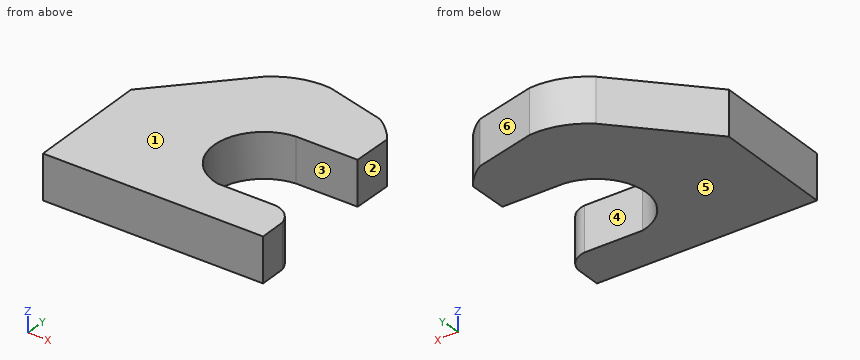
```python
from build123d import *

# Parameters (mm, degrees)
TABAN_FLAN_1_DEPTH         = 50
KES_EKSTR_ZYON1_DEPTH      = 585.997809561
KES_EKSTR_ZYON1_DEPTH_BACK = 585.997809561


# Sheet-metal steps are written as plain solids
with BuildPart() as part:
    # Çizim1 → Taban-Flanş1 (new body)
    with BuildSketch(Plane.XY):
        with BuildLine():
            Line((0, 0), (218.5, 0))
            ThreePointArc((218.5, 0), (276, 50), (333.5, 0))
            Line((333.5, 0), (360, 0))
            Line((360, 0), (449, 0))
            Line((449, 0), (458.997671741, 0.215777088))
            Line((458.997671741, 0.215777088), (455.997671741, 139.215777088))
            ThreePointArc((455.997671741, 139.215777088), (447.698955646, 153.213358252), (432.909011054, 160))
            Line((432.909011054, 160), (367.081412811, 160))
            ThreePointArc((367.081412811, 160), (323.554697394, 218.317011668), (374.513743955, 270.265297284))
            Line((374.513743955, 270.265297284), (434.798113421, 270.265297284))
            Line((434.798113421, 270.265297284), (444.798113421, 270.265297284))
            Line((444.798113421, 270.265297284), (444.798113421, 315.516988045))
            ThreePointArc((444.798113421, 315.516988045), (432.826102146, 329.550683033), (418.309236409, 340.931994828))
            Line((418.309236409, 340.931994828), (348.808103312, 358.867771111))
            ThreePointArc((348.808103312, 358.867771111), (316.270646866, 355.31487857), (287.772711056, 339.215910531))
            Line((287.772711056, 339.215910531), (171.828858079, 213.879290682))
            ThreePointArc((171.828858079, 213.879290682), (144.61514494, 194.164293468), (113.814091907, 180.726941422))
            ThreePointArc((113.814091907, 180.726941422), (82.931673061, 178.777598724), (53.149679292, 187.177395023))
            Line((53.149679292, 187.177395023), (53.149679292, 80.862415296))
            Line((53.149679292, 80.862415296), (0, 0))
        make_face()
    extrude(amount=TABAN_FLAN_1_DEPTH)

    # Çizim2 → Kes-Ekstrüzyon1 (cut, two sides: drawn at the far end of the back side and taken through both)
    with BuildSketch(Plane.XY.offset(50).offset(-KES_EKSTR_ZYON1_DEPTH_BACK)):
        with BuildLine():
            Line((456.658866876, 108.580402505), (206.600646856, 108.580402505))
            Line((206.600646856, 108.580402505), (203.587052823, 248.210259333))
            Line((203.587052823, 248.210259333), (171.828858079, 213.879290682))
            ThreePointArc((171.828858079, 213.879290682), (144.61514494, 194.164293468), (113.814091907, 180.726941422))
            ThreePointArc((113.814091907, 180.726941422), (82.931673061, 178.777598724), (53.149679292, 187.177395023))
            Line((53.149679292, 187.177395023), (53.149679292, 80.862415296))
            Line((53.149679292, 80.862415296), (0, 0))
            Line((0, 0), (218.5, 0))
            ThreePointArc((218.5, 0), (276, 50), (333.5, 0))
            Line((333.5, 0), (449, 0))
            Line((449, 0), (458.997671741, 0.215777088))
            Line((458.997671741, 0.215777088), (456.658866876, 108.580402505))
        make_face()
    extrude(amount=KES_EKSTR_ZYON1_DEPTH + KES_EKSTR_ZYON1_DEPTH_BACK, mode=Mode.SUBTRACT)


solid = part.part
```
Model file for the job. Use its own axes, mm. Face numbers are marked on the shaded views. A direction names the side the tool comes from. Give positions to 0.01 mm unless a question says otherwise; leave off trailing zeros. Loops run counter-clockwise (first coordinate to the right, second up) from the corner with the lowest first, then second, coordinate; pieces in that order, holes last. Notation, with made-up numbers: M 0.25,10 L 52.25,10 A21 cw 52.25,14 Z; hole C -14.5,14 d9. An arc over 180 degrees is marked long. Use one line per item in the form item = value.
Item 1: Slice it at C-C on x = 394.5. List the corners of the cut face in (y, z), and give its area (3 significant figures).
Filled in:
outline = M 108.58,0 L 160,0 L 160,50 L 108.58,50 Z; M 270.27,0 L 347.08,0 L 347.08,50 L 270.27,50 Z
area = 6,410 mm^2
Item 2: Slice it at B-B on z = 24.5. List the corners of the cut face in (x, y).
Filled in:
outline = M 203.59,248.21 L 206.6,108.58 L 456.66,108.58 L 456,139.22 A27.29 ccw 432.91,160 L 367.08,160 A55.92 cw 374.51,270.27 L 444.8,270.27 L 444.8,315.52 A92.57 ccw 418.31,340.93 L 348.81,358.87 A81.28 ccw 287.77,339.22 Z
Item 3: Slice it at A-A on x = 337.5. List the corners of the cut face in (y, z), and give its area (3 significant figures).
Filled in:
outline = M 108.58,0 L 177.47,0 L 177.47,50 L 108.58,50 Z; M 251.65,0 L 359.14,0 L 359.14,50 L 251.65,50 Z
area = 8,820 mm^2
Item 4: Slice it at D-D on y = 152.5. List the corners of the cut face in (x, z).
Filled in:
outline = M 205.65,0 L 448.46,0 L 448.46,50 L 205.65,50 Z
Item 5: Two-plate mould, pull along Y, no slides. Class the marked faces 4, 5 and 6: released by +Y, released by -Y, zero draft, split by the parting line, or undercut.
Filled in:
face_4 = undercut
face_5 = zero draft
face_6 = released by +Y
Item 6: Which spindle directions (+Z, -Z, +X, -X, +Y, -Y) get a long thin tool onto all of the face, cutting with end or side? Do the marked faces 1, 2 and 3. Say none if no direction does.
Filled in:
face_1 = +Z, +X, -X, +Y, -Y
face_2 = +Z, -Z, +X, +Y
face_3 = +Z, -Z, +X
Item 7: Flat gauge pins, fed straight in: pin 1 Ø1.5 at (y, z) = (203, 31) entering from +X; pin 2 Ø12 at (x, z) = (356, 35.5) entering from +Y; pin 3 Ø12 at (y, z) = (283.5, 25) entering from +X. Where does each tip first touch, or does it go through?
Filled in:
pin_1 = 324.8
pin_2 = 358.56
pin_3 = 444.8
Item 8: Drill centre lines: L1, parallel to Y at x = 357.5, z = 24; L2, parallel to Y at x = 395.5, z = 21; L3, parallel to Y at x = 321.5, z = 42.5. Where is each one in solid material? Low to high.
Filled in:
L1 = 108.58 to 163.08, 266.03 to 356.62
L2 = 108.58 to 160, 270.27 to 346.82
L3 = 108.58 to 356.81
